```python
from build123d import *

# Parameters (mm, degrees)
SKETCH_W   = 213.36
SKETCH_H   = 128.5
SKETCH_R   = 1.5
SKETCH_R_2 = 2.9
SKETCH_W_2 = 2.5
SKETCH_H_2 = 68
SKETCH_W_3 = 4
SKETCH_H_3 = 6.7
SKETCH_W_4 = 14.85
SKETCH_H_4 = 13.85
PAD_DEPTH  = 1.85


with BuildPart() as part:
    # Sketch → Pad (new body)
    with BuildSketch(Plane.XY):
        with Locations((106.68, 64.25)):
            Rectangle(SKETCH_W, SKETCH_H)
        with Locations((18.87, 109.54)):
            Circle(SKETCH_R, mode=Mode.SUBTRACT)
        with Locations((18.741513, 29.54)):
            Circle(SKETCH_R, mode=Mode.SUBTRACT)
        with Locations((51.141013, 29.54)):
            Circle(SKETCH_R, mode=Mode.SUBTRACT)
        with Locations((51.2695, 109.54)):
            Circle(SKETCH_R, mode=Mode.SUBTRACT)
        with Locations((83.540513, 29.54)):
            Circle(SKETCH_R, mode=Mode.SUBTRACT)
        with Locations((83.669, 109.54)):
            Circle(SKETCH_R, mode=Mode.SUBTRACT)
        with Locations((115.940013, 29.54)):
            Circle(SKETCH_R, mode=Mode.SUBTRACT)
        with Locations((116.0685, 109.54)):
            Circle(SKETCH_R, mode=Mode.SUBTRACT)
        with Locations((165.07, 37.25)):
            Circle(SKETCH_R_2, mode=Mode.SUBTRACT)
        with Locations((174.5, 37.25)):
            Circle(SKETCH_R_2, mode=Mode.SUBTRACT)
        with Locations((183.93, 37.25)):
            Circle(SKETCH_R_2, mode=Mode.SUBTRACT)
        with Locations((193.36, 37.25)):
            Circle(SKETCH_R_2, mode=Mode.SUBTRACT)
        with Locations((165.07, 25.3)):
            Circle(SKETCH_R_2, mode=Mode.SUBTRACT)
        with Locations((174.5, 25.3)):
            Circle(SKETCH_R_2, mode=Mode.SUBTRACT)
        with Locations((183.93, 25.3)):
            Circle(SKETCH_R_2, mode=Mode.SUBTRACT)
        with Locations((193.36, 25.3)):
            Circle(SKETCH_R_2, mode=Mode.SUBTRACT)
        with Locations((165.07, 13.35)):
            Circle(SKETCH_R_2, mode=Mode.SUBTRACT)
        with Locations((174.5, 13.35)):
            Circle(SKETCH_R_2, mode=Mode.SUBTRACT)
        with Locations((183.93, 13.35)):
            Circle(SKETCH_R_2, mode=Mode.SUBTRACT)
        with Locations((193.36, 13.35)):
            Circle(SKETCH_R_2, mode=Mode.SUBTRACT)
        with Locations((18.84522, 69.54)):
            Rectangle(SKETCH_W_2, SKETCH_H_2, mode=Mode.SUBTRACT)
        with Locations((51.24474, 69.54)):
            Rectangle(SKETCH_W_2, SKETCH_H_2, mode=Mode.SUBTRACT)
        with Locations((83.64426, 69.54)):
            Rectangle(SKETCH_W_2, SKETCH_H_2, mode=Mode.SUBTRACT)
        with Locations((116.04378, 69.54)):
            Rectangle(SKETCH_W_2, SKETCH_H_2, mode=Mode.SUBTRACT)
        with Locations((165.95529, 52.45)):
            Rectangle(SKETCH_W_3, SKETCH_H_3, mode=Mode.SUBTRACT)
        with Locations((175.025228, 52.416668)):
            Rectangle(SKETCH_W_3, SKETCH_H_3, mode=Mode.SUBTRACT)
        with Locations((184.095167, 52.383335)):
            Rectangle(SKETCH_W_3, SKETCH_H_3, mode=Mode.SUBTRACT)
        with Locations((193.165106, 52.350003)):
            Rectangle(SKETCH_W_3, SKETCH_H_3, mode=Mode.SUBTRACT)
        with Locations((142.433745, 102.767182)):
            Rectangle(SKETCH_W_4, SKETCH_H_4, mode=Mode.SUBTRACT)
        with Locations((142.16844, 81.118535)):
            Rectangle(SKETCH_W_4, SKETCH_H_4, mode=Mode.SUBTRACT)
        with Locations((142.250409, 32.762028)):
            Rectangle(SKETCH_W_4, SKETCH_H_4, mode=Mode.SUBTRACT)
        with Locations((142.392972, 57.432843)):
            Rectangle(SKETCH_W_4, SKETCH_H_4, mode=Mode.SUBTRACT)
    extrude(amount=PAD_DEPTH)


solid = part.part
```
Work out the finished part from the listing and answer in its coordinate system (mm). Give positions to 0.01 mm unless a question says otherwise; leave off trailing zeros. Loops run counter-clockwise (first coordinate to the right, second up) from the corner with the lowest first, then second, coordinate; pieces in that order, holes last. Notation, with made-up numbers: (6.5, -4) -> (42.5, -4) arc R22 ccw to (42.5, 33) -> close; hole circle Ø9 at (63, 34.25). An arc over 180 degrees is marked (long way). Write item = value, one per line. Start each with the question number.
(1) Find section A-A on y = 13.35. Give the vertices of the cut face in (x, z).
(2) Find section C-C on y = 106. Give the vertices of the cut face in (x, z).
(3) Find section B-B on y = 79. Give the vertices of the cut face in (x, z), and give its area (3 significant figures).
(4) Find the intervals of material crossed by probe 1 along X at (y, z) = (71, 0.25); probe 2 along Y at (x, z) = (18.87, 1.05); probe 3 along Y at (x, z) = (140, 1.6), in increasing order. Write a range as from..to.
(5) Find section D-D on z = 0.7. Give the number of separate pieces and of enclosed holes in the cut face, and give its area (3 significant figures).
(6) The mould has two halves that part along Y. Classify faces 1 (the cylindrical face through (177.18, 12.24, 0.91)), 2 (the cylindrical face through (191.22, 15.31, 0.91)), 3 (the flat face through (105, 65, 1.85)): +Y half, -Y half, draft (parallel to the pull), parting line (faces both ways), or undercut.
From the geometry:
q1.outline = (0, 0) -> (162.17, 0) -> (162.17, 1.85) -> (0, 1.85) -> close; (167.97, 0) -> (171.6, 0) -> (171.6, 1.85) -> (167.97, 1.85) -> close; (177.4, 0) -> (181.03, 0) -> (181.03, 1.85) -> (177.4, 1.85) -> close; (186.83, 0) -> (190.46, 0) -> (190.46, 1.85) -> (186.83, 1.85) -> close; (196.26, 0) -> (213.36, 0) -> (213.36, 1.85) -> (196.26, 1.85) -> close
q2.outline = (0, 0) -> (135.01, 0) -> (135.01, 1.85) -> (0, 1.85) -> close; (149.86, 0) -> (213.36, 0) -> (213.36, 1.85) -> (149.86, 1.85) -> close
q3.outline = (0, 0) -> (17.6, 0) -> (17.6, 1.85) -> (0, 1.85) -> close; (20.1, 0) -> (49.99, 0) -> (49.99, 1.85) -> (20.1, 1.85) -> close; (52.49, 0) -> (82.39, 0) -> (82.39, 1.85) -> (52.49, 1.85) -> close; (84.89, 0) -> (114.79, 0) -> (114.79, 1.85) -> (84.89, 1.85) -> close; (117.29, 0) -> (134.74, 0) -> (134.74, 1.85) -> (117.29, 1.85) -> close; (149.59, 0) -> (213.36, 0) -> (213.36, 1.85) -> (149.59, 1.85) -> close
q3.area = 349 mm^2
q4.probe_1 = 0..17.6, 20.1..49.99, 52.49..82.39, 84.89..114.79, 117.29..213.36
q4.probe_2 = 0..28.05, 31.03..35.54, 103.54..108.04, 111.04..128.5
q4.probe_3 = 0..25.84, 39.69..50.51, 64.36..74.19, 88.04..95.84, 109.69..128.5
q5.separate_pieces = 1
q5.enclosed_holes = 32
q5.area = 25,400 mm^2
q6.face_1 = undercut
q6.face_2 = undercut
q6.face_3 = draft
